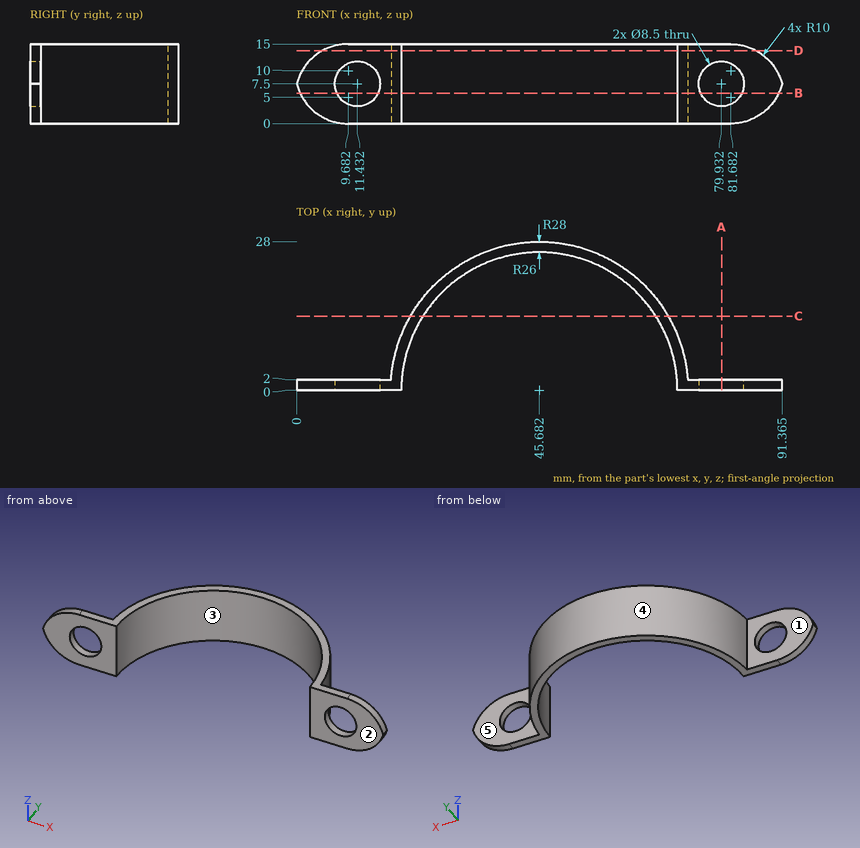
The drawing under review shows one solid part. Ordinate dimensions are in mm from its lowest x, y, z. A direction names the side the tool comes from. Give positions to 0.01 mm unless a question says otherwise; leave off trailing zeros. Write each loop counter-clockwise with the first axis right and the second up, starting at its lowest first coordinate (ties: lowest second). Pieces come first, ordered by that corner, then holes. Notation, with made-up numbers: (62.25, -1.5) -> (102.25, -1.5) arc R21 ccw to (102.25, 33.5) -> close; hole circle Ø4 at (53, 23). An arc over 180 degrees is marked (long way). Answer in a Markdown table with one row per item.
(1) Clearance check with flat-ended pins moving along their axes: pin 1 (5 mm diameter, centred on x = 77, z = 9, fed in from -Y); pin 2 (4 mm diameter, centred on x = 30, z = 9, fed in from +Y); pin 3 (4.5 mm diameter, centred on x = 81.5, z = 7, fed in from +Y); pin 4 (3 mm diameter, centred on x = 23.5, z = 7, fed in from -Y). State where each tip first meets the part, or that it passes through.
Results:
| item | result |
|---|---|
| pin 1 | y = 0 |
| pin 2 | y = 24.43 |
| pin 3 | through |
| pin 4 | y = 10.73 |
(2) To check wall thickness, follow probe 1 along Y at (x, z) = (86, 2); probe 2 along X at (y, z) = (20, 5.5) (1 decimal); probe 3 along X at (y, z) = (15.5, 12.5) (1 decimal). State the ranges of each line that lie inside material, in increasing order.
Results:
| item | result |
|---|---|
| probe 1 | 0 to 2 |
| probe 2 | 26.1 to 29.1, 62.3 to 65.3 |
| probe 3 | 22.4 to 24.8, 66.6 to 69 |
(3) Consider section B-B (z = 5.75). State the section outline as (x, y) points (1 decimal), then the cut area to 3 significant figures.
Results:
| item | result |
|---|---|
| outline | (0.6, 0) -> (7.6, 0) -> (7.6, 2) -> (0.6, 2) -> close; (15.3, 0) -> (19.7, 0) arc R26 cw to (71.7, 0) -> (76.1, 0) -> (76.1, 2) -> (73.6, 2) arc R28 ccw to (17.8, 2) -> (15.3, 2) -> close; (83.8, 0) -> (90.7, 0) -> (90.7, 2) -> (83.8, 2) -> close |
| area | 207 mm2 |
(4) Consider section D-D (z = 13.75). State the section outline as (x, y) points, then the cut area to 3 significant figures.
Results:
| item | result |
|---|---|
| outline | (4.84, 0) -> (19.68, 0) arc R26 cw to (71.68, 0) -> (86.52, 0) -> (86.52, 2) -> (73.61, 2) arc R28 ccw to (17.75, 2) -> (4.84, 2) -> close |
| area | 221 mm2 |
(5) Consider section C-C (y = 14). State the section outline as (x, z) points.
Results:
| item | result |
|---|---|
| outline | (21.43, 0) -> (23.77, 0) -> (23.77, 15) -> (21.43, 15) -> close; (67.59, 0) -> (69.93, 0) -> (69.93, 15) -> (67.59, 15) -> close |
(6) Consider section A-A (x = 80). State the section outline as (y, z) points, then the cut area to 3 significant figures.
Results:
| item | result |
|---|---|
| outline | (0, 0) -> (2, 0) -> (2, 3.25) -> (0, 3.25) -> close; (0, 11.75) -> (2, 11.75) -> (2, 15) -> (0, 15) -> close |
| area | 13.0 mm2 |
(7) Mouldability with a two-part tool opening along X and no side actions: class the marked faces 3, 4 and 5 as +X half, -X half, draft (parallel to the pull), parting line (faces both ways), or undercut.
Results:
| item | result |
|---|---|
| face 3 | undercut |
| face 4 | parting line |
| face 5 | draft |
(8) For the marked faces 1 and 2, list the 3-axis set-ups (+Z, -Z, +X, -X, +Y, -Y) from which the entire face can be reached by the end or side of a thin tool; tool diameter is ignored.
Results:
| item | result |
|---|---|
| face 1 | +Z, -Z, -X, +Y |
| face 2 | +Z, -Z, +X, -X, -Y |
